Build history of the part. All positions in model axes, mm. Round coordinates to 2 decimals unless told otherwise and drop trailing zeros. Loops run counter-clockwise (first coordinate to the right, second up) from the corner with the lowest first, then second, coordinate; pieces in that order, holes last.
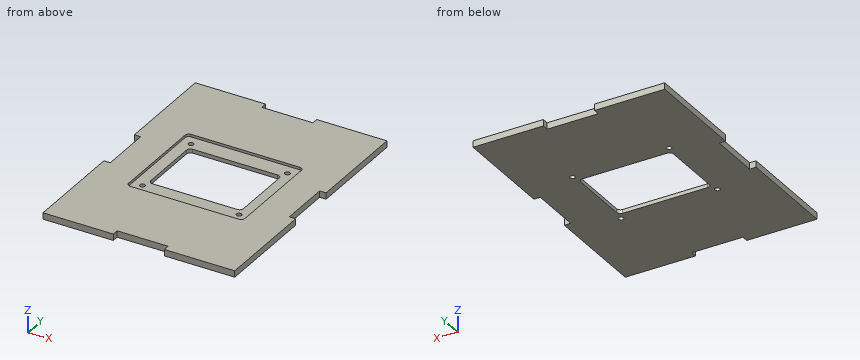
from build123d import *

# Parameters (mm, degrees)
CROQUIS1_W              = 150
CROQUIS1_H              = 200
SALIENTE_EXTRUIR1_DEPTH = 5
CROQUIS3_R              = 2
CROQUIS3_W              = 40
CROQUIS3_H              = 5
CROQUIS3_W_2            = 5
CROQUIS3_H_2            = 40
CROQUIS3_W_3            = 72.5
CROQUIS3_H_3            = 53
CORTAR_EXTRUIR2_DEPTH   = 5
CROQUIS4_W              = 91
CROQUIS4_H              = 80
CORTAR_EXTRUIR3_DEPTH   = 2
REDONDEO1_R             = 3


with BuildPart() as part:
    # Croquis1 → Saliente-Extruir1 (new body)
    with BuildSketch(Plane.XY):
        Rectangle(CROQUIS1_W, CROQUIS1_H)
    extrude(amount=SALIENTE_EXTRUIR1_DEPTH)

    # Croquis3 → Cortar-Extruir2 (cut)
    with BuildSketch(Plane.XY.offset(5)):
        with Locations((-37.75, 31.8)):
            Circle(CROQUIS3_R)
        with Locations((37.75, 31.8)):
            Circle(CROQUIS3_R)
        with Locations((37.75, -31.8)):
            Circle(CROQUIS3_R)
        with Locations((-37.75, -31.8)):
            Circle(CROQUIS3_R)
        with Locations((0, 97.5)):
            Rectangle(CROQUIS3_W, CROQUIS3_H)
        with Locations((0, -97.5)):
            Rectangle(CROQUIS3_W, CROQUIS3_H)
        with Locations((-72.5, 0)):
            Rectangle(CROQUIS3_W_2, CROQUIS3_H_2)
        with Locations((72.5, 0)):
            Rectangle(CROQUIS3_W_2, CROQUIS3_H_2)
        Rectangle(CROQUIS3_W_3, CROQUIS3_H_3)
    extrude(amount=-CORTAR_EXTRUIR2_DEPTH, mode=Mode.SUBTRACT)

    # Croquis4 → Cortar-Extruir3 (cut)
    with BuildSketch(Plane.XY.offset(5)):
        Rectangle(CROQUIS4_W, CROQUIS4_H)
    extrude(amount=-CORTAR_EXTRUIR3_DEPTH, mode=Mode.SUBTRACT)

    # Redondeo1
    redondeo1_edges = [part.edges().sort_by_distance(p)[0] for p in [
        (-45.5, -40, 4),
        (-45.5, 40, 4),
        (45.5, 40, 4),
        (45.5, -40, 4),
        (36.25, 26.5, 1.5),
        (36.25, -26.5, 1.5),
        (-36.25, -26.5, 1.5),
        (-36.25, 26.5, 1.5),
    ]]
    fillet(redondeo1_edges, radius=REDONDEO1_R)


solid = part.part
(1) Slice it at A-A on z = 2. Count the separate pieces of the cut face and the enclosed holes in it, plus the area to 3 significant figures.
Responses:
separate pieces: 1
enclosed holes: 5
area: 25,300 mm2
(2) Slice it at B-B on x = -25.5. List the corners of the cut face in (y, z), plus the area to 3 significant figures.
Responses:
outline: (-100, 0) - (-26.5, 0) - (-26.5, 3) - (-40, 3) - (-40, 5) - (-100, 5) - close; (26.5, 0) - (100, 0) - (100, 5) - (40, 5) - (40, 3) - (26.5, 3) - close
area: 681 mm2
(3) Pin check, flat tips, straight feed: P1, Ø5, axis at x = 37.75, y = -31.8, coming from the +Z side; P2, Ø1, axis at x = 13, z = 0.5, coming from the +Y side; P3, Ø2.5, axis at y = -2.5, z = 3.5, coming from the -X side. Stop position of each tip, or through.
Responses:
P1: stops at z = 3
P2: stops at y = 95
P3: stops at x = -70
(4) Probe line 1 (Y direction, x = -37.75, z = 0.9); line 2 (Y direction, x = 25, z = 3.8); line 3 (Y direction, x = -32, z = 1.7). List the from-to ranges inside material, lowest first.
Responses:
line 1: y = -100 to -33.8, -29.8 to 29.8, 33.8 to 100
line 2: y = -100 to -40, 40 to 100
line 3: y = -100 to -26.5, 26.5 to 100
(5) Slice it at C-C on x = 4.5. List the corners of the cut face in (y, z).
Responses:
outline: (-95, 0) - (-26.5, 0) - (-26.5, 3) - (-40, 3) - (-40, 5) - (-95, 5) - close; (26.5, 0) - (95, 0) - (95, 5) - (40, 5) - (40, 3) - (26.5, 3) - close
